Source: CAD feature listing. Evaluate the final solid. Frame: model axes, mm. A direction names the side the tool comes from. Give positions to 0.01 mm unless a question says otherwise; leave off trailing zeros. Order: outer loops, then holes, each group sorted by start corner. A loop starts at its lowest first (then second) coordinate and runs counter-clockwise, first axis right, second up. Notation, with made-up numbers: M 34,83.5 L 41,83.5 A7 cw 41,94.5 Z; hole C -15.75,84.25 d6. An arc over 180 degrees is marked long. One line per question, with ' | ' between items. Start each with the question number.
from build123d import *

# Parameters (mm, degrees)
F0_W     = 45
F0_H     = 45
F1_DEPTH = 442.5
F2_W     = 20
F2_H     = 45
F3_DEPTH = 20
F4_W     = 15
F4_H     = 45
F5_DEPTH = 20
F6_R     = 5


with BuildPart() as f1:
    # F0 (on Right) → F1 (new body, symmetric)
    with BuildSketch(Plane.YZ):
        Rectangle(F0_W, F0_H)
    extrude(amount=F1_DEPTH, both=True)

    # F2 (on face) → F3 (join)
    with BuildSketch(Plane.YZ.offset(442.5)):
        Rectangle(F2_W, F2_H)
    extrude(amount=F3_DEPTH)

    # F4 (on face) → F5 (join)
    with BuildSketch(Plane(origin=(-442.5, 0, 0), x_dir=(0, -1, 0), z_dir=(-1, 0, 0))):
        Rectangle(F4_W, F4_H)
    extrude(amount=F5_DEPTH)

    # F6
    f6_edges = [f1.edges().sort_by_distance(p)[0] for p in [
        (0, -22.5, 22.5),
        (0, 22.5, 22.5),
        (0, -22.5, -22.5),
        (0, 22.5, -22.5),
    ]]
    fillet(f6_edges, radius=F6_R)


solid = f1.part
Item 1: Line query: line 1 (Y direction, x = 362.5, z = -18); line 2 (X direction, y = -16.5, z = -4); line 3 (X direction, y = 8, z = 21.5). Output: solid intervals per line, ascending.
Item 2: Cut plane A-A on z = -10.5. Return the cut outline in (x, y).
Item 3: Pin query (flat end, axial travel): pin 1 Ø6 at (x, z) = (456.5, 10.5) entering from +Y; pin 2 Ø7.5 at (y, z) = (-18.5, 1) entering from -X; pin 3 Ø22 at (x, z) = (-451, -5) entering from +Y; pin 4 Ø16 at (x, z) = (-457, 7) entering from -Y. Return the tip coordinate at first contact, or that it passes through.
Item 4: Reachability of faces 1 (the flat face through (-452, 7.5, 0)), 2 (the flat face through (452, -10, 0)), 3 (the flat face through (-442.5, -15, 0)), 4 (the flat face through (452, 10, 0)) from +Z, -Z, +X, -X, +Y, -Y: full face, straight path, thin tool, end or side. Return the list, or none.
Results are:
1) line 1: y = -22.47 to 22.47 | line 2: x = -442.5 to 442.5 | line 3: x = -442.5 to 462.5
2) outline: M -462.5,-7.5 L -442.5,-7.5 L -442.5,-22.5 L 442.5,-22.5 L 442.5,-10 L 462.5,-10 L 462.5,10 L 442.5,10 L 442.5,22.5 L -442.5,22.5 L -442.5,7.5 L -462.5,7.5 Z
3) pin 1: stops at y = 10 | pin 2: stops at x = -442.5 | pin 3: stops at y = 22.5 | pin 4: stops at y = -7.5
4) face 1: +Z, -Z, -X, +Y | face 2: +Z, -Z, +X, -Y | face 3: +Z, -Z, -X, -Y | face 4: +Z, -Z, +X, +Y
